```python
from build123d import *

# Parameters (mm, degrees)
SKETCH1_R           = 1.524
SKETCH1_R_2         = 7.9375
SKETCH1_R_3         = 7.250000001
BOSS_EXTRUDE1_DEPTH = 6.35
SKETCH1_3_R         = 7.9375
SKETCH1_3_R_2       = 7.250000001
CUT_EXTRUDE1_DEPTH  = 4.699


with BuildPart() as part:
    # Sketch1 → Boss-Extrude1 (new body)
    # profile 1 of 2: a face of its own
    with BuildSketch(Plane.XY):
        with BuildLine():
            Line((387.508701588, 293.783854224), (363.858701588, 293.783854224))
            ThreePointArc((363.858701588, 293.783854224), (361.613637557, 292.853918255), (360.683701588, 290.608854224))
            Line((360.683701588, 290.608854224), (360.683701588, 243.958854223))
            ThreePointArc((360.683701588, 243.958854223), (361.613637557, 241.713790192), (363.858701588, 240.783854223))
            Line((363.858701588, 240.783854223), (387.508701588, 240.783854223))
            ThreePointArc((387.508701588, 240.783854223), (389.753765618, 241.713790192), (390.683701588, 243.958854223))
            Line((390.683701588, 243.958854223), (390.683701588, 290.608854224))
            ThreePointArc((390.683701588, 290.608854224), (389.753765618, 292.853918255), (387.508701588, 293.783854224))
        make_face()
        with Locations((386.478701588, 283.783854224)):
            Circle(SKETCH1_R, mode=Mode.SUBTRACT)
        with Locations((375.683701588, 283.783854224)):
            Circle(SKETCH1_R_2, mode=Mode.SUBTRACT)
        with BuildLine():
            ThreePointArc((382.133701588, 248.333854223), (384.683701589, 245.783854223), (387.233701589, 248.333854223))
            Line((387.233701589, 248.333854223), (387.233701589, 263.233854225))
            ThreePointArc((387.233701589, 263.233854225), (384.683701589, 265.783854225), (382.133701588, 263.233854225))
            Line((382.133701588, 263.233854225), (382.133701588, 248.333854223))
        make_face(mode=Mode.SUBTRACT)
        with BuildLine():
            ThreePointArc((369.233701587, 263.233854225), (366.683701588, 265.783854224), (364.133701589, 263.233854225))
            Line((364.133701589, 263.233854225), (364.133701589, 248.333854223))
            ThreePointArc((364.133701589, 248.333854223), (366.683701588, 245.783854224), (369.233701587, 248.333854223))
            Line((369.233701587, 248.333854223), (369.233701587, 263.233854225))
        make_face(mode=Mode.SUBTRACT)
    # profile 2 of 2: a face of its own
    with BuildSketch(Plane.XY):
        with Locations((375.683701588, 283.783854224)):
            Circle(SKETCH1_R_2)
        with Locations((375.683701588, 283.783854224)):
            Circle(SKETCH1_R_3, mode=Mode.SUBTRACT)
    extrude(amount=BOSS_EXTRUDE1_DEPTH)

    # Sketch1_3 → Cut-Extrude1 (cut)
    with BuildSketch(Plane.XY):
        with Locations((375.683701588, 283.783854224)):
            Circle(SKETCH1_3_R)
        with Locations((375.683701588, 283.783854224)):
            Circle(SKETCH1_3_R_2, mode=Mode.SUBTRACT)
    extrude(amount=CUT_EXTRUDE1_DEPTH, mode=Mode.SUBTRACT)


solid = part.part
```
Input: part model. Units: mm. Frame: model coordinates. A direction names the side the tool comes from. Give positions to 0.01 mm unless a question says otherwise; leave off trailing zeros. Order: outer loops, then holes, each group sorted by start corner. A loop starts at its lowest first (then second) coordinate and runs counter-clockwise, first axis right, second up. Notation, with made-up numbers: (80, -12.5) - (115, -12.5) arc R13 cw to (115, -0.5) - close; hole circle Ø2 at (-40, 25). An arc over 180 degrees is marked (long way). Put each result on its own line as item: value.
Item 1: Section query A-A, the plane y = 260. Return loops of the section in (x, z).
Found:
outline: (360.68, 0) - (364.13, 0) - (364.13, 6.35) - (360.68, 6.35) - close; (369.23, 0) - (382.13, 0) - (382.13, 6.35) - (369.23, 6.35) - close; (387.23, 0) - (390.68, 0) - (390.68, 6.35) - (387.23, 6.35) - close
Item 2: Draft query along Y for faces 4 (the flat face through (376, 293.784, 3)), 5 (the cylindrical face through (366.74, 265.783, 3.131)), 6 (the flat face through (390.684, 267, 3)). Return one class per face: +Y half, -Y half, draft (parallel to the pull), parting line (faces both ways), or undercut.
Found:
face 4: +Y half
face 5: undercut
face 6: draft
Item 3: Access query for faces 1 (the cylindrical face through (366.628, 245.784, 3.131)), 2 (the cylindrical face through (389.78, 292.83, 3.13)), 3 (the flat face through (379, 277, 4.699)). Directions: +Z, -Z, +X, -X, +Y, -Y. A direction counts if a zero-diameter tool reaches every point of the face in a straight line with its end or side. Return the directions, or none.
Found:
face 1: +Z, -Z
face 2: +Z, -Z, +X, +Y
face 3: -Z
Item 4: Section query B-B, the plane x = 367.25. Return loops of the section in (y, z), then the cut area to 3 significant figures.
Found:
outline: (240.78, 0) - (245.85, 0) - (245.85, 6.35) - (240.78, 6.35) - close; (265.72, 0) - (293.78, 0) - (293.78, 6.35) - (265.72, 6.35) - close
area: 210 mm^2
Item 5: Section query C-C, the plane z = 2. Count the separate pieces of the cut face and the enclosed holes in it, then the cut area to 3 significant figures.
Found:
separate pieces: 1
enclosed holes: 4
area: 1,180 mm^2
Item 6: Section query D-D, the plane y = 280. Return loops of the section in (x, z), then the cut area to 3 significant figures.
Found:
outline: (360.68, 0) - (368.71, 0) - (368.71, 4.7) - (369.5, 4.7) - (369.5, 6.35) - (360.68, 6.35) - close; (381.87, 4.7) - (382.66, 4.7) - (382.66, 0) - (390.68, 0) - (390.68, 6.35) - (381.87, 6.35) - close
area: 105 mm^2
Item 7: Ray query, L1, parallel to X at y = 251.5, z = 3; L2, parallel to X at y = 284, z = 3; L3, parallel to Y at x = 384.5, z = 2.5. Return the intervals inside material, ascending. Write a range as from..to.
Found:
L1: x = 360.68..364.13, 369.23..382.13, 387.23..390.68
L2: x = 360.68..367.75, 383.62..384.97, 387.99..390.68
L3: y = 240.78..245.79, 265.78..293.78
